Work out the finished part from the listing and answer in its coordinate system (mm). Round coordinates to 2 decimals unless told otherwise and drop trailing zeros. Loops run counter-clockwise (first coordinate to the right, second up) from the corner with the lowest first, then second, coordinate; pieces in that order, holes last. Notation, with made-up numbers: (-19, 29.25) -> (37, 29.25) arc R22 cw to (37, 41.25) -> close; hole circle Ø10 at (11.25, 26.25). An arc over 180 degrees is marked (long way). Write item = value, one per line. Start each with the question number.
```python
from build123d import *

# Parameters (mm, degrees)
SKETCH1_W                    = 419.1
SKETCH1_H                    = 533.4
SKETCH1_W_2                  = 246.0625
SKETCH1_H_2                  = 346.075
OVERALL_SHAPE_DEPTH          = 6.35
SKETCH5_W                    = 258.7625
SKETCH5_H                    = 358.775
GLASS_INSET_CUT_DEPTH        = 3.19999995
GLASS_INSET_FILLETS_R        = 1.27
FILLET1_R                    = 19.05
F_10_32_TAPPED_HOLE3_D       = 4.0386
F_10_32_TAPPED_HOLE3_DEPTH   = 6.35
F_10_32_TAPPED_HOLE7_D       = 4.0386
F_10_32_TAPPED_HOLE7_DEPTH   = 6.35
F_5_16_18_TAPPED_HOLE1_D     = 6.5278
F_5_16_18_TAPPED_HOLE1_DEPTH = 6.35


with BuildPart() as part:
    # Sketch1 → Overall shape (new body)
    with BuildSketch(Plane(origin=(0, 0, 0), x_dir=(1, 0, 0), z_dir=(0, 1, 0))):
        with Locations((209.55, 266.7)):
            Rectangle(SKETCH1_W, SKETCH1_H)
        with Locations((209.55, 271.4625)):
            Rectangle(SKETCH1_W_2, SKETCH1_H_2, mode=Mode.SUBTRACT)
    extrude(amount=OVERALL_SHAPE_DEPTH)

    # Sketch5 → Glass inset cut (cut)
    with BuildSketch(Plane(origin=(0, 6.35, 0), x_dir=(1, 0, 0), z_dir=(0, 1, 0))):
        with Locations((209.55, 271.4625)):
            Rectangle(SKETCH5_W, SKETCH5_H)
    extrude(amount=-GLASS_INSET_CUT_DEPTH, mode=Mode.SUBTRACT)

    # Glass inset fillets
    glass_inset_fillets_edges = [part.edges().sort_by_distance(p)[0] for p in [
        (80.16875, 4.750000025, -92.075),
        (80.16875, 4.750000025, -450.85),
        (338.93125, 4.750000025, -450.85),
        (338.93125, 4.750000025, -92.075),
    ]]
    fillet(glass_inset_fillets_edges, radius=GLASS_INSET_FILLETS_R)

    # Fillet1
    fillet1_edges = [part.edges().sort_by_distance(p)[0] for p in [
        (419.1, 3.175, 0),
        (0, 3.175, 0),
    ]]
    fillet(fillet1_edges, radius=FILLET1_R)

    # #10-32 Tapped Hole3
    with Locations(Plane(origin=(0, 6.35, 0), x_dir=(1, 0, 0), z_dir=(0, 1, 0))):
        with Locations((63.5, 469.9), (355.6, 469.9), (355.6, 63.5), (63.5, 63.5)):
            Hole(F_10_32_TAPPED_HOLE3_D / 2, depth=F_10_32_TAPPED_HOLE3_DEPTH)

    # #10-32 Tapped Hole7
    with Locations(Plane(origin=(0, 6.35, 0), x_dir=(1, 0, 0), z_dir=(0, 1, 0))):
        with Locations((22.479, 514.8707), (22.479, 452.8185), (396.621, 514.8707), (396.621, 452.8185)):
            Hole(F_10_32_TAPPED_HOLE7_D / 2, depth=F_10_32_TAPPED_HOLE7_DEPTH)

    # 5/16-18 Tapped Hole1
    with Locations(Plane(origin=(0, 6.35, 0), x_dir=(1, 0, 0), z_dir=(0, 1, 0))):
        with Locations((22.479, 276.7965), (22.479, 212.7504), (396.621, 276.7965), (396.621, 212.7504)):
            Hole(F_5_16_18_TAPPED_HOLE1_D / 2, depth=F_5_16_18_TAPPED_HOLE1_DEPTH)


solid = part.part
```
Item 1: Section B-B (z = -389) is taken. Determine the outline of the cut face in (x, y).
Item 2: Section C-C (y = 2) is taken. Count the separate pieces of the cut face and the enclosed holes in it, then the cut area to 3 significant figures.
Item 3: A flat-ended cylindrical pin translates along its axis: pin 1 (3 mm diameter, centred on x = 396.62, z = -452.82, fed in from +Y). Find the tip coordinate at first contact, or state that the pin passes through.
Item 4: Section A-A (x = 160) is taken. Determine the outline of the cut face in (y, z) (3 decimals), then the cut area to 3 significant figures.
Item 5: Find the intervals of material crossed by line 1 along X through (y, z) = (1.5, -469.9); line 2 along Z through (x, y) = (173, 1.5) (3 decimals); line 3 along Z through (x, y) = (116, 4.25) (3 decimals), in increasing order. Write a range as [from, to].
Item 6: The mould has two halves that part along X. Classify faces 1 (the flat face through (346, 6.35, -270)), 2 (the flat face through (209, 3.15, -445)), 3 (the cylindrical face through (413.37, 3.22, -5.43)): pulls with the +X half, pulls with the -X half, needs draft (parallel to the pull), parting line crosses it, or undercut.
Worked answers:
q1.outline = (0, 0) -> (86.52, 0) -> (86.52, 3.15) -> (80.17, 3.15) -> (80.17, 6.35) -> (0, 6.35) -> close; (332.58, 0) -> (419.1, 0) -> (419.1, 6.35) -> (338.93, 6.35) -> (338.93, 3.15) -> (332.58, 3.15) -> close
q2.separate_pieces = 1
q2.enclosed_holes = 13
q2.area = 138,000 mm2
q3.pin_1 = through
q4.outline = (0, -533.4) -> (6.35, -533.4) -> (6.35, -450.85) -> (3.15, -450.85) -> (3.15, -444.5) -> (0, -444.5) -> close; (0, -98.425) -> (3.15, -98.425) -> (3.15, -92.075) -> (6.35, -92.075) -> (6.35, 0) -> (0, 0) -> close
q4.area = 1,150 mm2
q5.line_1 = [0, 61.48], [65.52, 353.58], [357.62, 419.1]
q5.line_2 = [-533.4, -444.5], [-98.425, 0]
q5.line_3 = [-533.4, -450.85], [-92.075, 0]
q6.face_1 = needs draft
q6.face_2 = undercut
q6.face_3 = pulls with the +X half
